The listing builds one solid part. Answer for the finished solid, in the listing's coordinates (mm). Coordinates: 2 decimals unless noted, no trailing zeros. Loops run counter-clockwise (first coordinate to the right, second up) from the corner with the lowest first, then second, coordinate; pieces in that order, holes last. Notation, with made-up numbers: (43.25, 27.5) - (88.25, 27.5) arc R16 ccw to (88.25, 53.5) - close; hole circle Ø4 at (13.5, 35). An arc over 180 degrees is marked (long way). Return JSON: item names as keys, results as strings. Group by question number.
1. Find the intervals of material crossed by line 1 along Y through (x, z) = (4.5, 3.75); line 2 along Z through (x, y) = (79.5, 28); line 3 along Z through (x, y) = (3, 24.35), in increasing order.
2. Section A-A (x = 17) is taken. Write down the section's boundary in (y, z).
3. Each of these flat-tipped pins is pushed along its axis until it touches: P1, Ø0.9, axis at x = 1.5, z = 4, coming from the +Y side; P2, Ø0.6, axis at x = 6.5, z = 5, coming from the -Y side; P3, Ø17, axis at x = 59.5, y = 18, coming from the +Z side. Where does it stop, or does it pass through?
```python
from build123d import *

# Parameters (mm, degrees)
BOSS_EXTRUDE1_DEPTH     = 34
FILLET1_R               = 5
CUT_EXTRUDE1_DEPTH      = 2.7
CUT_EXTRUDE1_DEPTH_BACK = 2.7
SKETCH3_R               = 3
CUT_EXTRUDE2_DEPTH      = 2.5
CUT_EXTRUDE2_DEPTH_BACK = 2.5
CUT_EXTRUDE3_DEPTH      = 2.7
CUT_EXTRUDE3_DEPTH_BACK = 2.7
SKETCH6_R               = 3
SKETCH7_W               = 20.448170552
SKETCH7_H               = 9.707468646
CUT_EXTRUDE4_DEPTH      = 4
SKETCH8_W               = 21.500714273
SKETCH8_H               = 8.005332222
CUT_EXTRUDE5_DEPTH      = 4
CHAMFER1_SIZE           = 3
FILLET2_R               = 5
SKETCH9_W               = 5.495998252
SKETCH9_H               = 5.2
SKETCH9_W_2             = 5.526351164
CUT_EXTRUDE6_DEPTH      = 2


with BuildPart() as part:
    # Sketch1 → Boss-Extrude1 (new body)
    with BuildSketch(Plane(origin=(0, 0, 0), x_dir=(1, 0, 0), z_dir=(0, 1, 0))):
        with BuildLine():
            Line((85, 0), (3, 0))
            Line((3, 0), (3, -2))
            ThreePointArc((3, -2), (3.866025404, -2.127718677), (4.658312395, -2.5))
            Line((4.658312395, -2.5), (85, -2.5))
            Line((85, -2.5), (85, 0))
        make_face()
        with BuildLine():
            Line((3, -2), (3, 0))
            Line((3, 0), (0, 0))
            Line((0, 0), (0, -2.5))
            Line((0, -2.5), (1.341687605, -2.5))
            ThreePointArc((1.341687605, -2.5), (2.133974596, -2.127718677), (3, -2))
        make_face()
        with BuildLine():
            ThreePointArc((0, -5), (0.356617963, -3.581362835), (1.341687605, -2.5))
            Line((1.341687605, -2.5), (0, -2.5))
            Line((0, -2.5), (0, -5))
        make_face()
        with BuildLine():
            Line((3, -4.4), (3, -2.5))
            Line((3, -2.5), (0, -5))
            ThreePointArc((0, -5), (0.878679656, -7.121320344), (3, -8))
            Line((3, -8), (3, -5.6))
            ThreePointArc((3, -5.6), (2.4, -5), (3, -4.4))
        make_face()
        with BuildLine():
            Line((4.658312395, -2.5), (3, -2.5))
            Line((3, -2.5), (3, -4.4))
            ThreePointArc((3, -4.4), (3.424264069, -4.575735931), (3.6, -5))
            ThreePointArc((3.6, -5), (3.424264069, -5.424264069), (3, -5.6))
            Line((3, -5.6), (3, -8))
            ThreePointArc((3, -8), (5.121320344, -7.121320344), (6, -5))
            ThreePointArc((6, -5), (5.643382037, -3.581362835), (4.658312395, -2.5))
        make_face()
        with BuildLine():
            Line((0, -5), (3, -2.5))
            Line((3, -2.5), (1.341687605, -2.5))
            ThreePointArc((1.341687605, -2.5), (0.356617963, -3.581362835), (0, -5))
        make_face()
        with BuildLine():
            Line((3, -2.5), (3, -2))
            ThreePointArc((3, -2), (2.133974596, -2.127718677), (1.341687605, -2.5))
            Line((1.341687605, -2.5), (3, -2.5))
        make_face()
        with BuildLine():
            ThreePointArc((4.658312395, -2.5), (3.866025404, -2.127718677), (3, -2))
            Line((3, -2), (3, -2.5))
            Line((3, -2.5), (4.658312395, -2.5))
        make_face()
    extrude(amount=BOSS_EXTRUDE1_DEPTH)

    # Fillet1
    fillet1_edges = [part.edges().sort_by_distance(p)[0] for p in [
        (4.658312395, 17, 2.5),
    ]]
    fillet(fillet1_edges, radius=FILLET1_R)

    # Sketch3 → Cut-Extrude1 (cut, two sides: drawn at the far end of the back side and taken through both)
    with BuildSketch(Plane(origin=(0, 24, 0), x_dir=(1, 0, 0), z_dir=(0, 1, 0)).offset(-CUT_EXTRUDE1_DEPTH_BACK)):
        with Locations((3, -5)):
            Circle(SKETCH3_R)
    extrude(amount=CUT_EXTRUDE1_DEPTH + CUT_EXTRUDE1_DEPTH_BACK, mode=Mode.SUBTRACT)

    # Sketch5 → Cut-Extrude2 (cut, two sides: drawn at the far end of the back side and taken through both)
    with BuildSketch(Plane(origin=(0, 24, 0), x_dir=(1, 0, 0), z_dir=(0, 1, 0)).offset(-CUT_EXTRUDE2_DEPTH_BACK)):
        Polygon((3, -2), (-2.094466052, -2), (-2.094466052, -6.13547251), (2.720170219, -6.13547251), align=None)
    extrude(amount=CUT_EXTRUDE2_DEPTH + CUT_EXTRUDE2_DEPTH_BACK, mode=Mode.SUBTRACT)

    # Sketch6 → Cut-Extrude3 (cut, two sides: drawn at the far end of the back side and taken through both)
    with BuildSketch(Plane(origin=(0, 10, 0), x_dir=(1, 0, 0), z_dir=(0, 1, 0)).offset(-CUT_EXTRUDE3_DEPTH_BACK)):
        with Locations((3, -5)):
            Circle(SKETCH6_R)
        with BuildLine():
            ThreePointArc((0, -5), (0.878679656, -2.878679656), (3, -2))
            Line((3, -2), (0, -2))
            Line((0, -2), (0, -5))
        make_face()
    extrude(amount=CUT_EXTRUDE3_DEPTH + CUT_EXTRUDE3_DEPTH_BACK, mode=Mode.SUBTRACT)

    # Sketch7 → Cut-Extrude4 (cut)
    with BuildSketch(Plane(origin=(0, 34, 0), x_dir=(1, 0, 0), z_dir=(0, 1, 0))):
        with Locations((4.670623526, -7.353734323)):
            Rectangle(SKETCH7_W, SKETCH7_H)
    extrude(amount=-CUT_EXTRUDE4_DEPTH, mode=Mode.SUBTRACT)

    # Sketch8 → Cut-Extrude5 (cut)
    with BuildSketch(Plane.XZ):
        with Locations((3.718915286, 6.502666111)):
            Rectangle(SKETCH8_W, SKETCH8_H)
    extrude(amount=-CUT_EXTRUDE5_DEPTH, mode=Mode.SUBTRACT)

    # Chamfer1
    chamfer1_edges = [part.edges().sort_by_distance(p)[0] for p in [
        (0, 0, 1.25),
        (0, 34, 1.25),
    ]]
    chamfer(chamfer1_edges, length=CHAMFER1_SIZE)

    # Fillet2
    fillet2_edges = [part.edges().sort_by_distance(p)[0] for p in [
        (85, 34, 1.25),
        (85, 0, 1.25),
    ]]
    fillet(fillet2_edges, radius=FILLET2_R)

    # Sketch9 → Cut-Extrude6 (cut)
    with BuildSketch(Plane.XY.offset(5.9375)):
        with Locations((6.215533717, 9.9)):
            Rectangle(SKETCH9_W, SKETCH9_H)
        with Locations((5.763175582, 23.9)):
            Rectangle(SKETCH9_W_2, SKETCH9_H)
    extrude(amount=-CUT_EXTRUDE6_DEPTH, mode=Mode.SUBTRACT)


solid = part.part
```
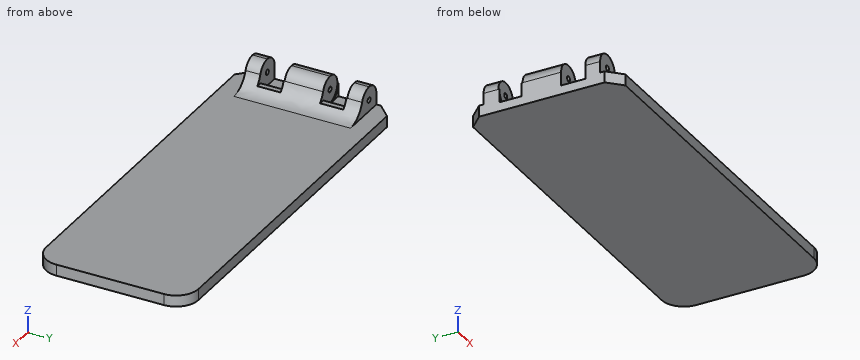
The answers:
{
 "1": {"line 1": "y = 4 to 7.3, 12.7 to 21.3, 26.7 to 30", "line 2": "z = 0 to 2.5", "line 3": "z = 0 to 2"},
 "2": {"outline": "(0, 0) - (34, 0) - (34, 2.5) - (0, 2.5) - close"},
 "3": {"P1": "stops at y = 30", "P2": "stops at y = 4", "P3": "stops at z = 2.5"}
}
